from build123d import *

# Parameters (mm, degrees)
F2_R     = 1.016
F3_R     = 1.524
F4_R     = 0.762
F6_DEPTH = 25.4
F8_D     = 2.9464


with BuildPart() as f1:
    # F0 (on Front) → F1 (revolve)
    with BuildSketch(Plane.XZ):
        Polygon((-17.4389516755, -9.398), (-36.0310370011, -9.398), (-36.0310370011, -12.7), (-21.8070370011, -12.7), (20.3569629989, -20.066), (20.3569629989, -29.21), (30.5169629989, -29.21), (30.5169629989, -27.31135), (25.0559629989, -27.31135), (25.0559629989, -16.891), align=None)
    revolve(axis=Axis((-0.3203684359, 0, 0), (1, 0, 0)))

    # F2
    f2_edges = [f1.edges().sort_by_distance(p)[0] for p in [
        (20.356963, 0, 29.21),
    ]]
    fillet(f2_edges, radius=F2_R)

    # F3
    f3_edges = [f1.edges().sort_by_distance(p)[0] for p in [
        (20.356963, 0, 20.066),
    ]]
    fillet(f3_edges, radius=F3_R)

    # F4
    f4_edges = [f1.edges().sort_by_distance(p)[0] for p in [
        (-36.031037, 0, 12.7),
    ]]
    fillet(f4_edges, radius=F4_R)

    # F5 (on Top) → F6 (cut, symmetric)
    with BuildSketch(Plane.XY):
        with BuildLine():
            ThreePointArc((-17.6282525063, 17.526), (-15.7683805668, 13.0358719395), (-11.2782525063, 11.176))
            Line((-11.2782525063, 11.176), (9.4349629989, 11.176))
            ThreePointArc((9.4349629989, 11.176), (13.9250910594, 13.0358719395), (15.7849629989, 17.526))
            Line((15.7849629989, 17.526), (15.7849629989, 21.3468402398))
            Line((15.7849629989, 21.3468402398), (-17.6282525063, 21.2479885668))
            Line((-17.6282525063, 21.2479885668), (-17.6282525063, 17.526))
        make_face()
        with BuildLine():
            Line((9.4349629989, -11.176), (-11.2782525063, -11.176))
            ThreePointArc((-11.2782525063, -11.176), (-15.7683805668, -13.0358719395), (-17.6282525063, -17.526))
            Line((-17.6282525063, -17.526), (-17.6282525063, -20.1750025153))
            Line((-17.6282525063, -20.1750025153), (15.7849629989, -21.3468402398))
            Line((15.7849629989, -21.3468402398), (15.7849629989, -17.526))
            ThreePointArc((15.7849629989, -17.526), (13.9250910594, -13.0358719395), (9.4349629989, -11.176))
        make_face()
    extrude(amount=F6_DEPTH, both=True, mode=Mode.SUBTRACT)

    # F8 (through all)
    with Locations(Plane.YZ.offset(25.0559629989)):
        with Locations((12.573, 21.7678), (21.7678, 12.573), (21.7678, -12.573), (12.573, -21.7678), (-12.573, -21.7678), (-21.7678, -12.573), (-21.7678, 12.573), (-12.573, 21.7678)):
            Hole(F8_D / 2)


solid = f1.part
Geometry check sheet. Reference: the model listing, model coordinates, mm. A direction names the side the tool comes from. Round coordinates to 2 decimals unless told otherwise and drop trailing zeros. Order: outer loops, then holes, each group sorted by start corner. A loop starts at its lowest first (then second) coordinate and runs counter-clockwise, first axis right, second up. Notation, with made-up numbers: M 54.5,27 L 108.5,27 A38 cw 108.5,65 Z; hole C -7.5,81.5 d7. An arc over 180 degrees is marked long. Write each question's results on one line, items separated by ' | '. Start each with the question number.
1. Draft check along Z on faces 4 (the face through (25.056, 13, -12)), 5 (the face through (22.674, 12.892, -23.206)), 6 (the face through (15.785, -18, 0)). Enter one of: pulls with the +Z half, pulls with the -Z half, needs draft (parallel to the pull), parting line crosses it, or undercut.
2. Set-up check for faces 1 (the face through (20.357, 18.9, 10.3)), 2 (the face through (-5.4, -11.176, 3.4)), 3 (the face through (15.785, 18, 0)): record each of +Z, -Z, +X, -X, +Y, -Y from which the full face is reachable in a straight line by a thin tool's end or side.
3. Material ranges on L1, parallel to X at y = 21, z = -10; L2, parallel to Y at x = 21, z = 2; L3, parallel to Z at x = 27, y = -13, recorded low to high. Write a range as from..to.
4. Go/stop test with flat-tipped pins: P1, Ø16.5, axis at x = -0.5, z = 1.5, coming from the -Y side; P2, Ø16.5, axis at x = -4.5, z = -2, coming from the +Y side; P3, Ø12, axis at y = -20, z = -15, coming from the -X side; P4, Ø10, axis at y = -10, z = -22.5, coming from the +X side. Record where each tip stops, or that it passes through.
5. Cross-section at A-A on y = 0. Record the boundary of the cut face in (x, z), plus the area to 3 significant figures.
6. Cross-section at B-B on x = -1. Record the boundary of the cut face in (y, z), plus the area to 3 significant figures.
7. Cross-section at C-C on z = 0. Give the number of separate pieces and of enclosed holes in the cut face, plus the area to 3 significant figures.
Resolved:
1) face 4: undercut | face 5: undercut | face 6: needs draft
2) face 1: -X | face 2: +Z, -Z, -Y | face 3: +Z, -Z, -X, +Y
3) L1: 20.36..25.06 | L2: -29.07..-16.05, 16.05..29.07 | L3: -26.16..-24.02, 24.02..26.16
4) P1: y = -11.18 | P2: y = 11.35 | P3: x = 15.07 | P4: x = 30.52
5) outline: M -36.03,-11.94 A0.76 ccw -35.27,-12.7 L -21.81,-12.7 L 19.1,-19.85 A1.52 cw 20.36,-21.35 L 20.36,-28.19 A1.02 ccw 21.37,-29.21 L 30.52,-29.21 L 30.52,-27.31 L 25.06,-27.31 L 25.06,-16.89 L -17.44,-9.4 L -36.03,-9.4 Z; M -36.03,9.4 L -17.44,9.4 L 25.06,16.89 L 25.06,27.31 L 30.52,27.31 L 30.52,29.21 L 21.37,29.21 A1.02 ccw 20.36,28.19 L 20.36,21.35 A1.52 cw 19.1,19.85 L -21.81,12.7 L -35.27,12.7 A0.76 ccw -36.03,11.94 Z | area: 571 mm2
6) outline: M -11.18,-11.91 A16.33 ccw 11.18,-11.91 L 11.18,-5.13 A12.3 cw -11.18,-5.13 Z; M -11.18,5.13 A12.3 cw 11.18,5.13 L 11.18,11.91 A16.33 ccw -11.18,11.91 Z | area: 209 mm2
7) separate pieces: 4 | enclosed holes: 0 | area: 335 mm2
